Verification items for the finished model (mm, model axes). A direction names the side the tool comes from. Give positions to 0.01 mm unless a question says otherwise; leave off trailing zeros. Write each loop counter-clockwise with the first axis right and the second up, starting at its lowest first coordinate (ties: lowest second). Pieces come first, ordered by that corner, then holes. Notation, with made-up numbers: (-31.5, -22.75) -> (9.5, -22.75) arc R21 ccw to (9.5, 12.25) -> close; hole circle Ø10 at (78.25, 60.5). An arc over 180 degrees is marked (long way). Write item = value, one per line.
from build123d import *

# Parameters (mm, degrees)
SKETCH2_W                       = 42.3
SKETCH2_H                       = 130
SKETCH2_R                       = 12.5
SKETCH2_R_2                     = 4.1
BOSS_EXTRUDE1_DEPTH             = 6.35
TAP_DRILL_FOR_M3X0_5_TAP1_D     = 2.5
TAP_DRILL_FOR_M3X0_5_TAP1_DEPTH = 21.15
TAP_DRILL_FOR_M3X0_5_TAP1_TIP   = 0.751075774
M3_CLEARANCE_HOLE1_D            = 3.4
F_1_4_CLEARANCE_HOLE1_D         = 6.7564
BOSS_EXTRUDE2_DEPTH             = 6.35
M4_CLEARANCE_HOLE1_D            = 4.5


with BuildPart() as part:
    # Sketch2 → Boss-Extrude1 (new body)
    with BuildSketch(Plane.XY):
        with Locations((0, 43.85)):
            Rectangle(SKETCH2_W, SKETCH2_H)
        Circle(SKETCH2_R, mode=Mode.SUBTRACT)
        with Locations((0, 25)):
            Circle(SKETCH2_R_2, mode=Mode.SUBTRACT)
        with Locations((0, 50)):
            Circle(SKETCH2_R_2, mode=Mode.SUBTRACT)
    extrude(amount=BOSS_EXTRUDE1_DEPTH)

    # Tap Drill for M3x0.5 Tap1
    with Locations(Plane(origin=(21.15, 0, 0), x_dir=(0, 0, 1), z_dir=(1, 0, 0))):
        with Locations((3.175, -50), (3.175, 0), (3.175, -25)):
            Hole(TAP_DRILL_FOR_M3X0_5_TAP1_D / 2, depth=TAP_DRILL_FOR_M3X0_5_TAP1_DEPTH)
            with Locations((0, 0, -(TAP_DRILL_FOR_M3X0_5_TAP1_DEPTH + TAP_DRILL_FOR_M3X0_5_TAP1_TIP / 2))):  # 118° drill point
                Cone(0, TAP_DRILL_FOR_M3X0_5_TAP1_D / 2, TAP_DRILL_FOR_M3X0_5_TAP1_TIP, mode=Mode.SUBTRACT)

    # M3 Clearance Hole1 (through all)
    with Locations(Plane.XY.offset(6.35)):
        with Locations((-15.5, 15.5), (-15.5, -15.5), (15.5, -15.5), (15.5, 15.5)):
            Hole(M3_CLEARANCE_HOLE1_D / 2)

    # 1/4 Clearance Hole1 (through all)
    with Locations(Plane.XY.offset(6.35)):
        with Locations((-13.15, 86.85), (-13.15, 100.85)):
            Hole(F_1_4_CLEARANCE_HOLE1_D / 2)

    # Sketch13 → Boss-Extrude2 (add)
    with BuildSketch(Plane.XY.offset(6.35)):
        Polygon((-21.15, 8.85), (-51.15, 26.170508076), (-51.15, 76.170508076), (-21.15, 93.491016151), align=None)
    extrude(amount=-BOSS_EXTRUDE2_DEPTH)

    # M4 Clearance Hole1 (through all)
    with Locations(Plane.XY.offset(6.35)):
        with Locations((-45.15, 59.170508076), (-21.15, 59.170508076), (-21.15, 43.170508076), (-45.15, 43.170508076)):
            Hole(M4_CLEARANCE_HOLE1_D / 2)


solid = part.part
Item 1: Mould release check, pull along Z, two halves, no side actions. Record for faces 1 (the cylindrical face through (12.41, 48.76, 3.34)), 2 (the flat face through (-7, 45, 0)), 3 (the cylindrical face through (12.41, 26.22, 3.45)), 4 (the flat face through (0, -21.15, 3)): +Z half, -Z half, draft (parallel to the pull), parting line (faces both ways), or undercut.
Response values:
face_1 = undercut
face_2 = -Z half
face_3 = undercut
face_4 = draft
Item 2: Material ranges on line 1 (Y direction, x = -46, z = 1.25); line 2 (Y direction, x = 0, z = 3.5); line 3 (Z direction, x = 17, y = 50) (3 decimals), recorded low to high.
Response values:
line_1 = 23.2 to 41.09, 45.25 to 57.09, 61.25 to 79.14
line_2 = -21.15 to -12.5, 12.5 to 20.9, 29.1 to 45.9, 54.1 to 108.85
line_3 = 0 to 1.925, 4.425 to 6.35
Item 3: Sectioned sample at C-C on z = 3. Give the number of separate pieces and of enclosed holes in the cut face, then the cut area to 3 significant figures.
Response values:
separate_pieces = 1
enclosed_holes = 10
area = 6,640 mm^2
Item 4: Sectioned sample at A-A on y = 50. Record the cut outline in (x, z) (3 decimals).
Response values:
outline = (-51.15, 0) -> (-4.1, 0) -> (-4.1, 6.35) -> (-51.15, 6.35) -> close; (4.1, 0) -> (21.15, 0) -> (21.15, 1.925) -> (4.1, 1.925) -> close; (4.1, 4.425) -> (21.15, 4.425) -> (21.15, 6.35) -> (4.1, 6.35) -> close
Item 5: Sectioned sample at D-D on x = -1. Record the cut outline in (y, z), then the cut area to 3 significant figures.
Response values:
outline = (-21.15, 0) -> (-12.46, 0) -> (-12.46, 6.35) -> (-21.15, 6.35) -> close; (12.46, 0) -> (21.02, 0) -> (21.02, 6.35) -> (12.46, 6.35) -> close; (28.98, 0) -> (46.02, 0) -> (46.02, 6.35) -> (28.98, 6.35) -> close; (53.98, 0) -> (108.85, 0) -> (108.85, 6.35) -> (53.98, 6.35) -> close
area = 566 mm^2
Item 6: Sectioned sample at B-B on y = 86.85. Record the cut outline in (x, z), then the cut area to 3 significant figures.
Response values:
outline = (-32.65, 0) -> (-16.53, 0) -> (-16.53, 6.35) -> (-32.65, 6.35) -> close; (-9.77, 0) -> (21.15, 0) -> (21.15, 6.35) -> (-9.77, 6.35) -> close
area = 299 mm^2
Item 7: Go/stop test with flat-tipped pins: P1, Ø9.5, axis at x = 0, y = 25, coming from the +Z side; P2, Ø1.5, axis at y = 25, z = 3.175, coming from the +X side; P3, Ø3, axis at y = 0, z = 3.175, coming from the -X side; P4, Ø1.5, axis at x = -34, z = 3, coming from the -Y side. Record where each tip stops, or that it passes through.
Response values:
P1 = 6.35
P2 = -4.03
P3 = -21.15
P4 = 15.84
Item 8: Set-up check for faces 5 (the flat face through (-21.15, 101, 3)), 6 (the cylindrical face through (-12.7, 90.2, 3.1)), 7 (the flat face through (-21.15, -6, 3)): record each of +Z, -Z, +X, -X, +Y, -Y from which the full face is reachable in a straight line by a thin tool's end or side.
Response values:
face_5 = +Z, -Z, -X, +Y
face_6 = +Z, -Z
face_7 = +Z, -Z, -X, -Y
